The figure shows three views and two pictorial views of one solid part (mm, origin at its lowest corner). Answer the questions. A direction names the side the tool comes from. Coordinates: 2 decimals unless noted, no trailing zeros. Loops run counter-clockwise (first coordinate to the right, second up) from the corner with the lowest first, then second, coordinate; pieces in that order, holes last. Notation, with made-up numbers: (20.25, -26.75) - (48.25, -26.75) arc R12 cw to (48.25, -10.75) - close; hole circle Ø1 at (-27, 46). An arc over 180 degrees is marked (long way). Write each question's results on one line, items separated by ' | '. Start each with the question number.
Item 1: Each of these flat-tipped pins is pushed along its axis until it touches: pin 1 Ø12 at (y, z) = (9, 19.5) entering from -X; pin 2 Ø1.5 at (x, y) = (70.5, 19) entering from +Z; pin 3 Ø5.5 at (y, z) = (6.5, 37) entering from +X. Where does it stop, or does it pass through?
Item 2: A tool of negligible diameter and unlimited length cuts with its end or side. For the marked faces 1, 2 and 3, from which of +Z, -Z, +X, -X, +Y, -Y can it reach the whole face along a straight path? Write none if from no direction.
Item 3: Section A-A, the plane y = 6 is taken. Write down the section's boundary in (x, z).
Item 4: Section C-C, the plane x = 74 is taken. Write down the section's boundary in (y, z), plus the area to 3 significant figures.
Item 5: Section B-B, the plane z = 35 is taken. Write down the section's boundary in (x, y), plus the area to 3 significant figures.
Item 6: Consider probe 1 along X at (y, z) = (8.75, 12.5); probe 2 along X at (y, z) = (19.5, 33.5); probe 3 along Z at (x, y) = (119.5, 4). Determine where each line is inside the solid, lowest interval first. Write a range as [from, to].
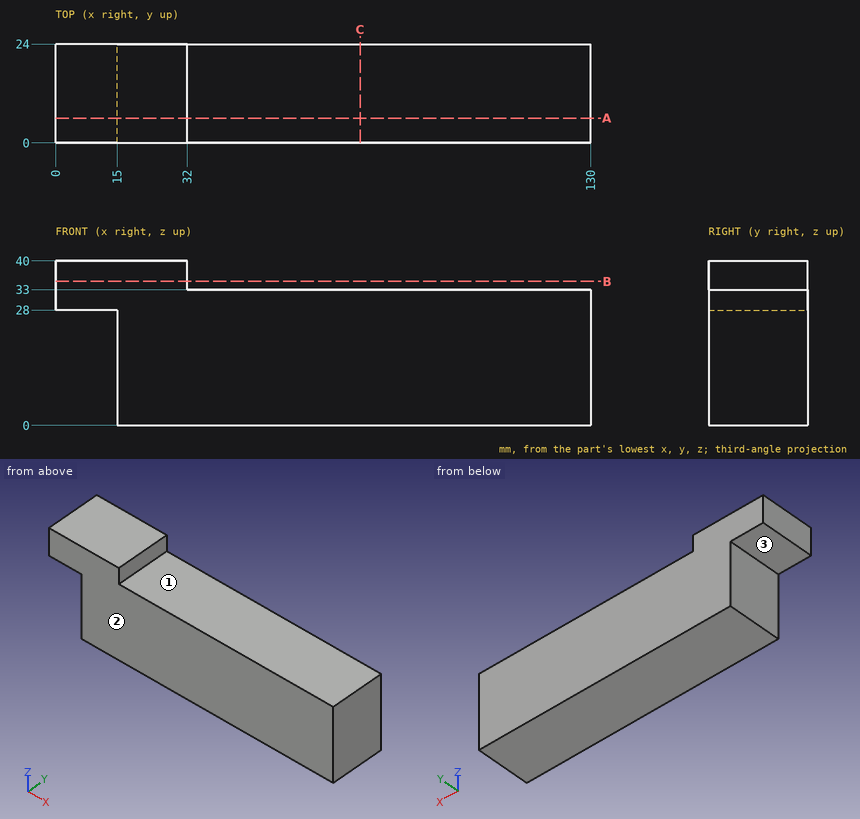
Answer key:
1) pin 1: stops at x = 15 | pin 2: stops at z = 33 | pin 3: stops at x = 32
2) face 1: +Z, +X, +Y, -Y | face 2: +Z, -Z, +X, -X, -Y | face 3: -Z, -X, +Y, -Y
3) outline: (0, 28) - (15, 28) - (15, 0) - (130, 0) - (130, 33) - (32, 33) - (32, 40) - (0, 40) - close
4) outline: (0, 0) - (24, 0) - (24, 33) - (0, 33) - close | area: 792 mm^2
5) outline: (0, 0) - (32, 0) - (32, 24) - (0, 24) - close | area: 768 mm^2
6) probe 1: x = [15, 130] | probe 2: x = [0, 32] | probe 3: z = [0, 33]
